The figure shows three views and two pictorial views of one solid part (mm, origin at its lowest corner). Answer the questions. Coordinates: 2 decimals unless noted, no trailing zeros. Order: outer loops, then holes, each group sorted by start corner. A loop starts at its lowest first (then second) coordinate and runs counter-clockwise, first axis right, second up. Notation, with made-up numbers: (17, 69) -> (52, 69) arc R25 ccw to (52, 88) -> close; hole circle Ø7 at (19, 12.25). An arc over 180 degrees is marked (long way). Use one line per item in the form item = value.
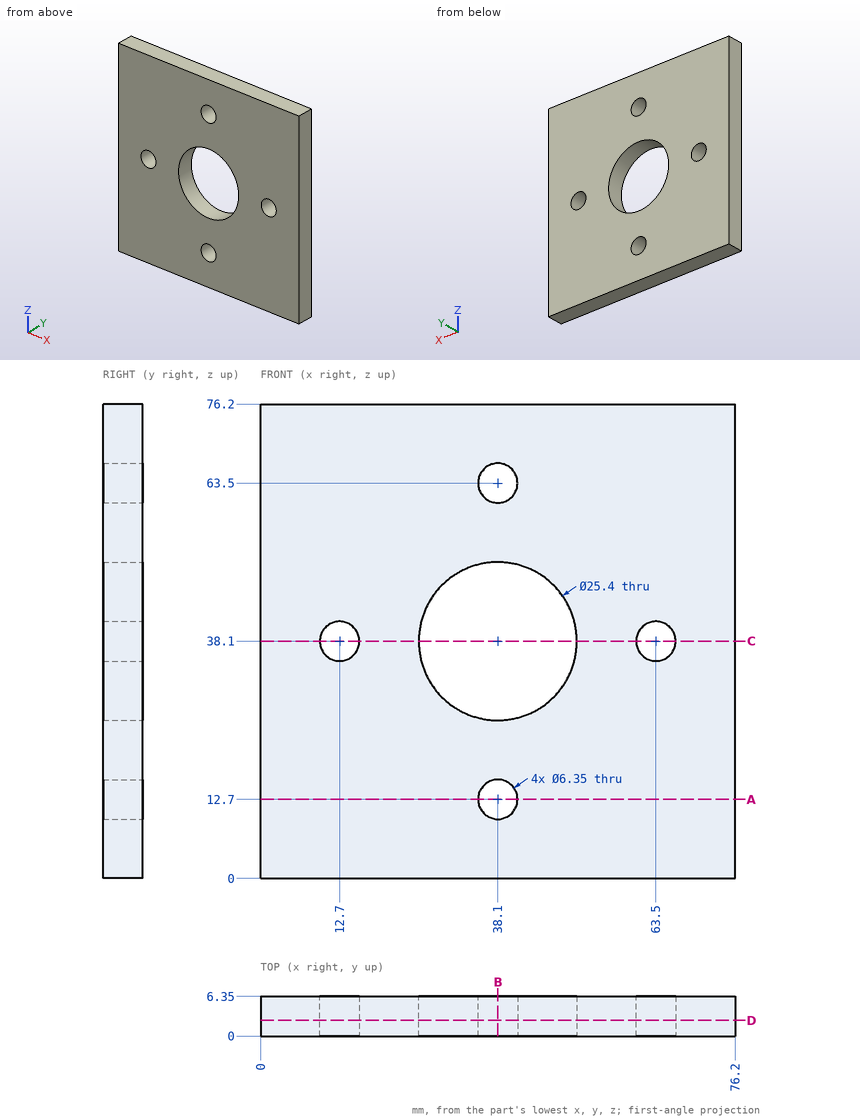
(1) This flat-tipped pin is pushed along its axis until it touches: P1, Ø5.5, axis at x = 12.7, z = 38.1, coming from the -Y side. Where does it stop, or does it pass through?
Data:
P1 = through
(2) Section B-B on x = 38.1 is taken. Write down the section's boundary in (y, z) (3 decimals).
Data:
outline = (0, 0) -> (6.35, 0) -> (6.35, 9.525) -> (0, 9.525) -> close; (0, 15.875) -> (6.35, 15.875) -> (6.35, 25.4) -> (0, 25.4) -> close; (0, 50.8) -> (6.35, 50.8) -> (6.35, 60.325) -> (0, 60.325) -> close; (0, 66.675) -> (6.35, 66.675) -> (6.35, 76.2) -> (0, 76.2) -> close
(3) Section C-C on z = 38.1 is taken. Write down the section's boundary in (x, y) (3 decimals), plus the area to 3 significant figures.
Data:
outline = (0, 0) -> (9.525, 0) -> (9.525, 6.35) -> (0, 6.35) -> close; (15.875, 0) -> (25.4, 0) -> (25.4, 6.35) -> (15.875, 6.35) -> close; (50.8, 0) -> (60.325, 0) -> (60.325, 6.35) -> (50.8, 6.35) -> close; (66.675, 0) -> (76.2, 0) -> (76.2, 6.35) -> (66.675, 6.35) -> close
area = 242 mm²
(4) Section A-A on z = 12.7 is taken. Write down the section's boundary in (x, y) (3 decimals), plus the area to 3 significant figures.
Data:
outline = (0, 0) -> (34.925, 0) -> (34.925, 6.35) -> (0, 6.35) -> close; (41.275, 0) -> (76.2, 0) -> (76.2, 6.35) -> (41.275, 6.35) -> close
area = 444 mm²
(5) Section D-D on y = 2.5 is taken. Write down the section's boundary in (x, z) (3 decimals).
Data:
outline = (0, 0) -> (76.2, 0) -> (76.2, 76.2) -> (0, 76.2) -> close; hole circle Ø6.35 at (12.7, 38.1); hole circle Ø25.4 at (38.1, 38.1); hole circle Ø6.35 at (38.1, 12.7); hole circle Ø6.35 at (38.1, 63.5); hole circle Ø6.35 at (63.5, 38.1)
(6) Straight lines are drawn through the part: line 1 along Z through (x, y) = (38.1, 2.25) (3 decimals); line 2 along Z through (x, y) = (12.7, 1.5) (3 decimals); line 3 along Z through (x, y) = (36.5, 3.75). For each, find the intervals that lie inside material, in ascending order.
Data:
line_1 = 0 to 9.525, 15.875 to 25.4, 50.8 to 60.325, 66.675 to 76.2
line_2 = 0 to 34.925, 41.275 to 76.2
line_3 = 0 to 9.96, 15.44 to 25.5, 50.7 to 60.76, 66.24 to 76.2
